Geometry: final body of the model. Coordinates: model frame, mm. Face numbers are marked on the shaded views. Round coordinates to 2 decimals unless told otherwise and drop trailing zeros. Write each loop counter-clockwise with the first axis right and the second up, starting at its lowest first coordinate (ties: lowest second). Pieces come first, ordered by that corner, then holes. Notation, with made-up numbers: M 47.25,-31.75 L 66.25,-31.75 A21 cw 66.25,-0.75 Z; hole C 26,15 d11. An arc over 180 degrees is marked long. Answer as CSV lines item,"result". Start each with the question number.
Q1. Mould query, pull axis X, two halves, no side actions, for the marked faces 1, 2 and 3. Classes: pulls with the +X half, pulls with the -X half, needs draft (parallel to the pull), parting line crosses it, or undercut.
Q2. Section query C-C on z = 21. Output: boundary loops of the cut face in (x, y), and give its area (3 significant figures).
Q3. Section query B-B on x = -2. Output: boundary loops of the cut face in (y, z).
Q4. Ray query, probe 1 along Z at (x, y) = (4.3, 0); probe 2 along Z at (x, y) = (-3, -2); probe 3 along X at (y, z) = (-1, 16). Return the intervals inside material, ascending.
Q5. First-contact query: pin 1 (5 mm diameter, centred on y = 3.5, z = 21.5, fed in from -X); pin 2 (4 mm diameter, centred on x = -3.5, y = 0, fed in from +Z). Flat tips, straight axial feed; report the tip coordinate or a pass-through.
Q6. Section query D-D on x = 1.5. Output: boundary loops of the cut face in (y, z), and give its area (3 significant figures).
```python
from build123d import *

# Parameters (mm, degrees)
F0_W     = 12
F0_H     = 10
F1_DEPTH = 5
F2_W     = 5.7338950146
F2_H     = 10
F3_DEPTH = 20
F4_R     = 1.6
F5_DEPTH = 10
F6_R     = 1.6
F7_DEPTH = 10
F8_R     = 4.99999


# Not quite as in the source:
# - a fillet or chamfer is up to 0.001 mm smaller than in the source, because OpenCascade refuses the exact size


with BuildPart() as f1:
    # F0 (on Top) → F1 (new body)
    with BuildSketch(Plane.XY):
        Rectangle(F0_W, F0_H)
    extrude(amount=F1_DEPTH)

    # F2 (on face) → F3 (join)
    with BuildSketch(Plane.XY.offset(5)):
        with Locations((3.1330524927, 0)):
            Rectangle(F2_W, F2_H)
    extrude(amount=F3_DEPTH)

    # F4 (on face) → F5 (cut)
    with BuildSketch(Plane(origin=(0.2661049854, 0, 0), x_dir=(0, -1, 0), z_dir=(-1, 0, 0))):
        with Locations((0, 21)):
            Circle(F4_R)
    extrude(amount=-F5_DEPTH, mode=Mode.SUBTRACT)

    # F6 (on face) → F7 (cut)
    with BuildSketch(Plane.XY.offset(5)):
        with Locations((-2, 0)):
            Circle(F6_R)
    extrude(amount=-F7_DEPTH, mode=Mode.SUBTRACT)

    # F8 (radius 5 in the source; OpenCascade refuses exactly that, so slightly less here)
    f8_edges = [f1.edges().sort_by_distance(p)[0] for p in [
        (-6, -5, 2.5),
        (-6, 5, 2.5),
    ]]
    fillet(f8_edges, radius=F8_R)


solid = f1.part
```
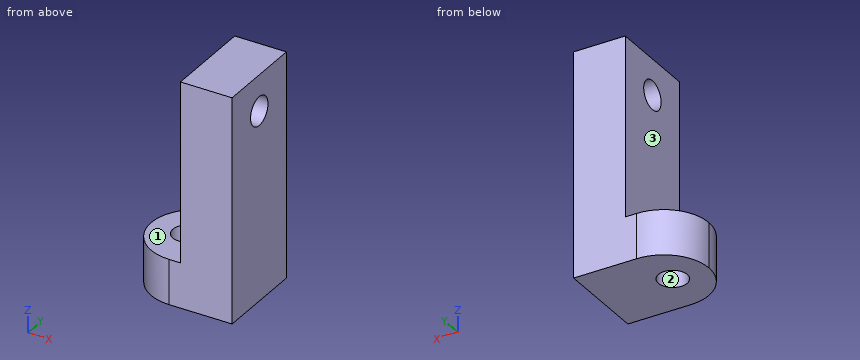
Entries:
1,face 1,"needs draft"
1,face 2,"undercut"
1,face 3,"pulls with the -X half"
2,outline,"M 0.27,-5 L 6,-5 L 6,-1.6 L 0.27,-1.6 Z; M 0.27,1.6 L 6,1.6 L 6,5 L 0.27,5 Z"
2,area,"39.0 mm^2"
3,outline,"M -4.9,0 L -1.6,0 L -1.6,5 L -4.9,5 Z; M 1.6,0 L 4.9,0 L 4.9,5 L 1.6,5 Z"
4,probe 1,"z = 0 to 19.4, 22.6 to 25"
4,probe 2,"z = 0 to 5"
4,probe 3,"x = 0.27 to 6"
5,pin 1,"stops at x = 0.27"
5,pin 2,"stops at z = 5"
6,outline,"M -5,0 L 5,0 L 5,25 L -5,25 Z; hole C 0,21 d3.2"
6,area,"242 mm^2"
